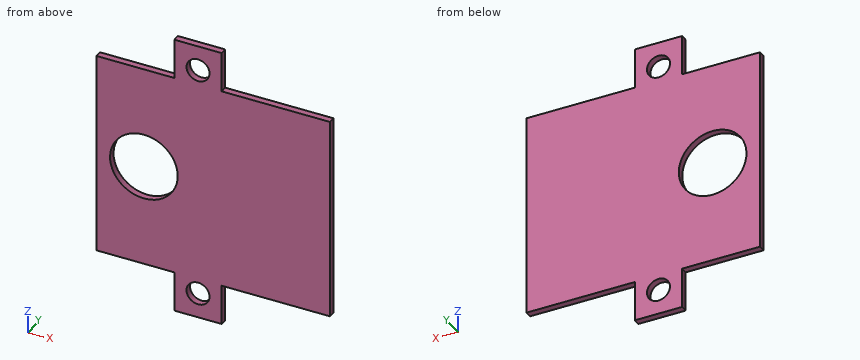
Autodesk Inventor part; units mm, degrees
ref_plane "YZ Plane" through (0, 0, 0) normal (1, 0, 0) x (0, 1, 0)
ref_plane "XZ Plane" through (0, 0, 0) normal (0, 1, 0) x (-1, 0, 0)
ref_plane "XY Plane" through (0, 0, 0) normal (0, 0, 1) x (1, 0, 0)
sketch "Sketch1" plane through (0, 0, 0) normal (0, 1, 0) x (-1, 0, 0)
  line L0 (8.0078, 6.9217) -> (-26.4922, 6.9217)
  line L1 (-26.4922, 6.9217) -> (-26.4922, -23.5583)
  line L2 (-26.4922, -23.5583) -> (8.0078, -23.5583)
  line L3 (8.0078, -23.5583) -> (8.0078, 6.9217)
  point P0 (0, 0)
  dimension "d0" = 34.5
  dimension "d1" = 30.48
extrude "Extrusion1" add sketch "Sketch1" along normal blind 1
sketch "Sketch2" plane through (0, 1, 0) normal (0, 1, 0) x (1, 0, 0)
  line L0 (-8.0078, 23.5583) -> (-8.0078, -6.9217)
  line L1 (-8.0078, -6.9217) -> (-8.0078, -5.9217)
  line L2 (-8.0078, -5.9217) -> (-7.0078, -5.9217)
  line L3 (26.4922, -6.9217) -> (26.4922, 23.5583)
  line L4 (26.4922, 23.5583) -> (26.4922, 22.5583)
  line L5 (26.4922, 22.5583) -> (25.4922, 22.5583)
  line L6 (-7.0078, -5.9217) -> (25.4922, -5.9217)
  line L7 (25.4922, -5.9217) -> (25.4922, 22.5583)
  line L8 (25.4922, 22.5583) -> (-7.0078, 22.5583)
  line L9 (-7.0078, 22.5583) -> (-7.0078, -5.9217)
  line L10 (-8.0078, 23.5583) -> (-8.0078, -6.9217)
  line L11 (-8.0078, -6.9217) -> (26.4922, -6.9217)
  line L12 (26.4922, -6.9217) -> (26.4922, 23.5583)
  line L13 (26.4922, 23.5583) -> (-8.0078, 23.5583)
  point P0 (0, 0)
  dimension "d4" = 1
  dimension "d5" = 1
  dimension "d6" = 1
  dimension "d7" = 1
extrude "Extrusion2" add sketch "Sketch2" along normal blind 2 contours L13 L3 L5 L8 L9 L2 L0 | L2 L6 L7 L5 L3 L11 L0
sketch "Sketch3" plane through (0, 0, 0) normal (0, 1, 0) x (1, 0, 0)
  line L0 (-7.0078, -5.9217) -> (-7.0078, 22.5583)
  line L1 (-7.0078, 8.3183) -> (6.9922, 8.3183)
  line L2 (6.9922, 8.3183) -> (6.9922, 25.8183)
  line L3 (6.9922, 25.8183) -> (6.9922, -9.1817)
  circle A0 centre (6.9922, -9.1817) radius 1.7
  circle A1 centre (6.9922, 25.8183) radius 1.7
  line L4 (25.4922, -5.9217) -> (-7.0078, -5.9217)
  line L5 (6.9922, -5.9217) -> (3.4922, -5.9217)
  line L6 (3.4922, -5.9217) -> (3.4922, -12.9217)
  line L7 (3.4922, -12.9217) -> (10.4922, -12.9217)
  line L8 (10.4922, -12.9217) -> (10.4922, -5.9217)
  line L9 (-7.0078, 22.5583) -> (25.4922, 22.5583)
  line L10 (3.4922, 22.5583) -> (3.4922, 29.5583)
  line L11 (3.4922, 29.5583) -> (10.4922, 29.5583)
  line L12 (10.4922, 29.5583) -> (10.4922, 22.5583)
  point P0 (0, 0)
  point P1 (9.2422, 22.5583)
  dimension "d10" = 14
  dimension "d11" = 17.5
  dimension "d12" = 35
  dimension "d13" = 3.4
  dimension "d14" = 3.4
  dimension "d15" = 3.5
  dimension "d16" = 7
  dimension "d17" = 7
  dimension "d18" = 7
  dimension "d31" = 7
extrude "Extrusion3" add sketch "Sketch3" along normal blind 1 contours L4 L8 L7 L6 | L10 L11 L12 L9
sketch "Sketch4" plane through (0, 1, 0) normal (0, 1, 0) x (1, 0, 0)
  line L0 (-7.0078, -5.9217) -> (-7.0078, 22.5583)
  line L1 (-7.0078, 8.3183) -> (-1.0078, 8.3183)
  point P0 (0, 0)
  dimension "d21" = 6
hole "Hole1" at (-1.0078, 1, -8.3183) direction (0, -1, 0) diameter 10 end through all
sketch "Sketch5" plane through (0, 3, 0) normal (0, 1, 0) x (1, 0, 0)
  line L0 (26.4922, 23.5583) -> (-8.0078, 23.5583)
  line L1 (-8.0078, 23.5583) -> (-8.0078, -6.9217)
  line L2 (-8.0078, -6.9217) -> (26.4922, -6.9217)
  line L3 (26.4922, -6.9217) -> (26.4922, 23.5583)
  line L4 (-7.0078, 22.5583) -> (25.4922, 22.5583)
  line L5 (25.4922, 22.5583) -> (25.4922, -5.9217)
  line L6 (25.4922, -5.9217) -> (-7.0078, -5.9217)
  line L7 (-7.0078, -5.9217) -> (-7.0078, 22.5583)
  point P0 (0, 0)
extrude "Extrusion4" cut sketch "Sketch5" against normal blind 2
properties part number "lid 4.0"
Verification items for the finished model (mm, model axes). Round coordinates to 2 decimals unless told otherwise and drop trailing zeros. Write each loop counter-clockwise with the first axis right and the second up, starting at its lowest first coordinate (ties: lowest second). Pieces come first, ordered by that corner, then holes. Notation, with made-up numbers: (58.25, -28) - (109.25, -28) arc R23 ccw to (109.25, 11) - close; hole circle Ø9 at (42.25, -7). An arc over 180 degrees is marked (long way). Answer as a JSON object with one key per item and string values. Group by question number.
Q1. Section check A-A, the plane z = -9.5. Enter the section's corners in (x, y), plus the area to 3 significant figures.
Q2. Section check D-D, the plane y = 0.5. Enter the section's corners in (x, z), plus the area to 3 significant figures.
Q3. Section check B-B, the plane x = 3. Enter the section's corners in (y, z).
Q4. Thickness scan on line 1 (X direction, y = 0.2, z = 9); line 2 (X direction, y = 0.1, z = -28); line 3 (Z direction, x = 3, y = 0.4). Record the ranges inside material, lowest first.
Q5. Go/stop test with flat-tipped pins: pin 1 Ø0.5 at (y, z) = (0.5, -28) entering from +X; pin 2 Ø0.5 at (y, z) = (0.5, -27.5) entering from -X; pin 3 Ø4.5 at (x, z) = (6.99, -25.82) entering from -Y; pin 4 Ø0.5 at (x, y) = (15, 0.5) entering from +Z. Record where each tip stops, or that it passes through.
Q6. Section check C-C, the plane x = 6.5. Enter the section's corners in (y, z), plus the area to 3 significant figures.
Found:
{
 "1": {"outline": "(-8.01, 0) - (-5.87, 0) - (-5.87, 1) - (-8.01, 1) - close; (3.85, 0) - (26.49, 0) - (26.49, 1) - (3.85, 1) - close", "area": "24.8 mm^2"},
 "2": {"outline": "(-8.01, -23.56) - (3.49, -23.56) - (3.49, -29.56) - (10.49, -29.56) - (10.49, -23.56) - (26.49, -23.56) - (26.49, 6.92) - (10.49, 6.92) - (10.49, 12.92) - (3.49, 12.92) - (3.49, 6.92) - (-8.01, 6.92) - close; hole circle Ø10 at (-1.01, -8.32); hole circle Ø3.4 at (6.99, -25.82); hole circle Ø3.4 at (6.99, 9.18)", "area": "1,040 mm^2"},
 "3": {"outline": "(0, -23.56) - (1, -23.56) - (1, -11.31) - (0, -11.31) - close; (0, -5.33) - (1, -5.33) - (1, 6.92) - (0, 6.92) - close"},
 "4": {"line 1": "x = 3.49 to 5.3, 8.68 to 10.49", "line 2": "x = 3.49 to 10.49", "line 3": "z = -23.56 to -11.31, -5.33 to 6.92"},
 "5": {"pin 1": "stops at x = 10.49", "pin 2": "stops at x = 3.49", "pin 3": "stops at y = 0", "pin 4": "stops at z = 6.92"},
 "6": {"outline": "(0, -29.56) - (1, -29.56) - (1, -27.45) - (0, -27.45) - close; (0, -24.19) - (1, -24.19) - (1, 7.55) - (0, 7.55) - close; (0, 10.81) - (1, 10.81) - (1, 12.92) - (0, 12.92) - close", "area": "36.0 mm^2"}
}
